Work out the finished part from the listing and answer in its coordinate system (mm). A direction names the side the tool comes from. Round coordinates to 2 decimals unless told otherwise and drop trailing zeros. Order: outer loops, then holes, each group sorted by start corner. A loop starts at its lowest first (then second) coordinate and runs counter-clockwise, first axis right, second up. Notation, with made-up numbers: (-25.5, 32.5) -> (12.5, 32.5) arc R28 ccw to (12.5, 59.5) -> close; hole circle Ø8 at (-29.75, 33). An arc over 180 degrees is marked (long way). Use one line per item in the form item = value.
Autodesk Inventor part; units mm, degrees
ref_plane "YZ Plane" through (0, 0, 0) normal (1, 0, 0) x (0, 1, 0)
ref_plane "XZ Plane" through (0, 0, 0) normal (0, 1, 0) x (-1, 0, 0)
ref_plane "XY Plane" through (0, 0, 0) normal (0, 0, 1) x (1, 0, 0)
sketch "Sketch1" plane through (0, 0, 0) normal (0, 1, 0) x (-1, 0, 0)
  line L0 (0, 0) -> (32, 0)
  line L1 (16, 0) -> (29, 0)
  circle A0 centre (29, 3) radius 1.375
  line L2 (16, 0) -> (16, 4.375)
  circle A1 centre (3, 3) radius 1.375
  line L3 (0, 0) -> (0, 6)
  line L4 (0, 6) -> (0, 11)
  line L5 (0, 11) -> (32, 11)
  line L6 (32, 11) -> (32, 0)
  dimension "d3" = 2.75
  dimension "d4" = 6
  dimension "d5" = 5
extrude "Extrusion1" add sketch "Sketch1" along normal blind 3
sketch "Sketch2" plane through (0, 3, 0) normal (0, 1, 0) x (1, 0, 0)
  line L0 (-32, -11) -> (0, -11)
  line L1 (0, -11) -> (0, 0)
  line L2 (-32, -11) -> (0, -11)
  line L3 (0, -11) -> (0, -6)
  line L4 (0, -6) -> (-32, -6)
  line L5 (-32, -6) -> (-32, -11)
  dimension "d8" = 5
extrude "Extrusion2" add sketch "Sketch2" along normal blind 29.5
sketch "Sketch3" plane through (0, 32.5, 0) normal (0, 1, 0) x (1, 0, 0)
  circle A0 centre (-3, -3) radius 1.375
  line L0 (-3, -3) -> (-3, -11)
  line L1 (-32, -11) -> (0, -11)
  line L2 (-3, -11) -> (-3, -15.4)
  circle A1 centre (-29, -3) radius 1.375
  line L3 (-29, -3) -> (-29, -11)
  line L4 (-29, -11) -> (-29, -15.4)
  circle A2 centre (-29, -15.4) radius 1.375
  circle A3 centre (-3, -15.4) radius 1.375
  line L5 (-3, -15.4) -> (-3, -41.4)
  circle A4 centre (-3, -41.4) radius 1.375
  circle A5 centre (-29, -41.4) radius 1.375
  line L6 (0, -6) -> (-32, -6)
  line L7 (-32, -6) -> (0, -6)
  line L8 (0, -6) -> (0, -45.8)
  line L9 (0, -45.8) -> (-32, -45.8)
  line L10 (-32, -45.8) -> (-32, -6)
  point P0 (0, 0)
  dimension "d11" = 4.4
  dimension "d12" = 2.75
  dimension "d13" = 26
  dimension "d14" = 39.8
extrude "Extrusion3" add sketch "Sketch3" along normal blind 3 contours L6 L8 L1 L0 | L0 L1 L3 L6 | L1 L8 L9 L10 | L3 L1 L10 L6
sketch "Sketch4" plane through (0, 35.5, 0) normal (0, 1, 0) x (1, 0, 0)
  circle A0 centre (-3, -15.4) radius 1.375
  circle A1 centre (-29, -41.4) radius 1.375
  circle A2 centre (-29, -15.4) radius 1.375
  circle A3 centre (-3, -41.4) radius 1.375
  circle A4 centre (-16, -28.4) radius 11.5
  point P0 (0, 0)
  dimension "d17" = 23
extrude "Extrusion4" cut sketch "Sketch4" against normal blind 3 contours A4
properties part number "Motor_Mount"
Item 1: The part is cut by section A-A, the plane z = 28.4. Give the vertices of the cut face in (x, y).
Findings:
outline = (-32, 32.5) -> (-27.5, 32.5) -> (-27.5, 35.5) -> (-32, 35.5) -> close; (-4.5, 32.5) -> (0, 32.5) -> (0, 35.5) -> (-4.5, 35.5) -> close
Item 2: The part is cut by section D-D, the plane x = -16. Give the vertices of the cut face in (y, z), and give its area (3 significant figures).
Findings:
outline = (0, 0) -> (3, 0) -> (3, 6) -> (35.5, 6) -> (35.5, 16.9) -> (32.5, 16.9) -> (32.5, 11) -> (0, 11) -> close; (32.5, 39.9) -> (35.5, 39.9) -> (35.5, 45.8) -> (32.5, 45.8) -> close
area = 231 mm^2
Item 3: The part is cut by section B-B, the plane x = -3. Give the vertices of the cut face in (y, z) (3 decimals), and give its area (3 significant figures).
Findings:
outline = (0, 0) -> (3, 0) -> (3, 1.625) -> (0, 1.625) -> close; (0, 4.375) -> (3, 4.375) -> (3, 6) -> (35.5, 6) -> (35.5, 14.025) -> (32.5, 14.025) -> (32.5, 11) -> (0, 11) -> close; (32.5, 16.775) -> (35.5, 16.775) -> (35.5, 40.025) -> (32.5, 40.025) -> close; (32.5, 42.775) -> (35.5, 42.775) -> (35.5, 45.8) -> (32.5, 45.8) -> close
area = 275 mm^2
Item 4: Determine the mould class of faces 1 (the cylindrical face through (-27.626, 1.479, 2.94)), 2 (the flat face through (-16, 1, 0)), 3 (the flat face through (-16, 34, 45.8)) for opening direction Z: released by +Z, released by -Z, zero draft, split by the parting line, or undercut.
Findings:
face_1 = undercut
face_2 = released by -Z
face_3 = released by +Z
Item 5: The part is cut by section C-C, the plane z = 15.4. Give the vertices of the cut face in (x, y) (3 decimals).
Findings:
outline = (-32, 32.5) -> (-30.375, 32.5) -> (-30.375, 35.5) -> (-32, 35.5) -> close; (-27.625, 32.5) -> (-4.375, 32.5) -> (-4.375, 35.5) -> (-27.625, 35.5) -> close; (-1.625, 32.5) -> (0, 32.5) -> (0, 35.5) -> (-1.625, 35.5) -> close
Item 6: For faces 4 (the flat face through (-16, 3, 3)), 5 (the flat face through (-16, 0, 6)), 6 (the flat face through (-16, 16, 11)), determine the directions among +Z, -Z, +X, -X, +Y, -Y from which every point of the face is accessible in a straight line to the end or side of a thin tool.
Findings:
face_4 = -Z, +X, -X, +Y
face_5 = +Z, -Z, +X, -X, -Y
face_6 = +Z, +X, -X, -Y
Item 7: Consider line 1 along Z through (x, y) = (-3, 33.85) (3 decimals); line 2 along Z through (x, y) = (-16, 33.9); line 3 along X through (y, z) = (33, 41). Determine where each line is inside the solid, lowest interval first.
Findings:
line_1 = 6 to 14.025, 16.775 to 40.025, 42.775 to 45.8
line_2 = 6 to 16.9, 39.9 to 45.8
line_3 = -32 to -30.32, -27.68 to -4.32, -1.68 to 0
Item 8: Flat-ended cylindrical pins translate along their axes: P1, Ø1.6, axis at x = -3, z = 15.4, coming from the +Y side; P2, Ø2, axis at x = -13.5, z = 39, coming from the -Y side; P3, Ø16, axis at x = -15.5, y = 11.5, coming from the +Z side; P4, Ø3.5, axis at x = -29, z = 3, coming from the +Y side. Find the tip coordinate at first contact, or state that the pin passes through.
Findings:
P1 = through
P2 = 32.5
P3 = 11
P4 = 3
